Verification items for the finished model (mm, model axes). A direction names the side the tool comes from. Coordinates: 2 decimals unless noted, no trailing zeros. Order: outer loops, then holes, each group sorted by start corner. A loop starts at its lowest first (then second) coordinate and runs counter-clockwise, first axis right, second up. Notation, with made-up numbers: M 24.25,48.25 L 63.25,48.25 A7 cw 63.25,53.25 Z; hole C -19.75,4.5 d2. An arc over 180 degrees is marked long. Answer as a JSON object with one key per item and string values. Group by question number.
(1) Cross-section at D-D (y = 25). Enter the section's corners in (x, z), plus the area to 3 significant figures.
(2) Cross-section at C-C (z = 12.5). Enter the section's corners in (x, y), plus the area to 3 significant figures.
(3) Material ranges on line 1 (X direction, y = 0, z = 13.25); line 2 (Y direction, x = 0, z = 19.25); line 3 (X direction, y = -31.5, z = 22), recorded low to high.
(4) Cross-section at B-B (y = 0). Enter the section's corners in (x, z), plus the area to 3 significant figures.
(5) Cross-section at A-A (x = 0). Enter the section's corners in (y, z).
(6) Gauge pin test, flat ends, axial feed: pin 1 Ø0.8 at (y, z) = (-27, 22) entering from +X; pin 2 Ø4 at (x, y) = (-2, -31.5) entering from +Z. Record the tip position at first contact, or that the pin passes through.
(7) Mould release check, pull along Z, two halves, no side actions. Record for faces 4 (the face through (-32, 1, 25)), 5 (the face through (-63.5, -1, 12)), 6 (the face through (30.304, -0.533, 22.496)), 7 (the face through (38, -1, 19.92)): released by +Z, released by -Z, zero draft, split by the parting line, or undercut.
(8) Access from +Z, -Z, +X, -X, +Y, -Y to the whole of each face (thin tool, end or side, straight path). Record for faces 1 (the face through (-1, -38.1, 12)), 2 (the face through (68.509, -0.992, 20.055)), 3 (the face through (-54.61, -1, 22)).
from build123d import *

# Parameters (mm, degrees)
F0_W     = 127
F0_H     = 76.2
F0_R     = 20
F1_DEPTH = 25
F2_W     = 6.35
F2_H     = 76.2
F3_DEPTH = 5.08
F5_DEPTH = 76.201
F6_R     = 7.62
F7_DEPTH = 12.7
F8_R     = 2.54
F9_SIZE  = 2.54


with BuildPart() as f1:
    # F0 (on Top) → F1 (new body)
    with BuildSketch(Plane.XY):
        Rectangle(F0_W, F0_H)
        Circle(F0_R, mode=Mode.SUBTRACT)
    extrude(amount=F1_DEPTH)

    # F2 (on face) → F3 (cut)
    with BuildSketch(Plane.XY.offset(25)):
        with Locations((-57.785, 0)):
            Rectangle(F2_W, F2_H)
        with BuildLine():
            Line((-6.35, -18.9651654356), (-6.35, -38.1))
            Line((-6.35, -38.1), (6.35, -38.1))
            Line((6.35, -38.1), (6.35, -18.9651654356))
            ThreePointArc((6.35, -18.9651654356), (0, -20), (-6.35, -18.9651654356))
        make_face()
        with BuildLine():
            Line((6.35, 38.1), (-6.35, 38.1))
            Line((-6.35, 38.1), (-6.35, 18.9651654356))
            ThreePointArc((-6.35, 18.9651654356), (0, 20), (6.35, 18.9651654356))
            Line((6.35, 18.9651654356), (6.35, 38.1))
        make_face()
    extrude(amount=-F3_DEPTH, mode=Mode.SUBTRACT)

    # F4 (on face) → F5 (cut, through all)
    with BuildSketch(Plane.XZ.offset(38.1)):
        Polygon((44.45, 25), (31.75, 25), (28.8170606325, 19.92), (47.3829393675, 19.92), align=None)
    extrude(amount=-F5_DEPTH, mode=Mode.SUBTRACT)

    # F6 (on face) → F7 (join)
    with BuildSketch(Plane.YZ.offset(63.5)):
        with Locations((0, 12.5)):
            Circle(F6_R)
    extrude(amount=F7_DEPTH)

    # F8
    f8_edges = [f1.edges().sort_by_distance(p)[0] for p in [
        (-6.35, -28.532583, 25),
        (-6.35, 28.532583, 25),
        (6.35, 28.532583, 25),
        (6.35, -28.532583, 25),
    ]]
    fillet(f8_edges, radius=F8_R)

    # F9
    f9_edges = [f1.edges().sort_by_distance(p)[0] for p in [
        (76.2, -7.62, 12.5),
    ]]
    chamfer(f9_edges, length=F9_SIZE)


solid = f1.part
Taken from the geometry:
{
 "1": {"outline": "M -63.5,0 L 63.5,0 L 63.5,25 L 44.45,25 L 47.38,19.92 L 28.82,19.92 L 31.75,25 L 8.89,25 A2.54 ccw 6.35,22.46 L 6.35,19.92 L -6.35,19.92 L -6.35,22.46 A2.54 ccw -8.89,25 L -54.61,25 L -54.61,19.92 L -60.96,19.92 L -60.96,25 L -63.5,25 Z", "area": "3,000 mm²"},
 "2": {"outline": "M -63.5,-38.1 L 63.5,-38.1 L 63.5,-7.62 L 73.66,-7.62 L 76.2,-5.08 L 76.2,5.08 L 73.66,7.62 L 63.5,7.62 L 63.5,38.1 L -63.5,38.1 Z; hole C 0,0 d40", "area": "8,610 mm²"},
 "3": {"line 1": "x = -63.5 to -20, 20 to 76.2", "line 2": "y = -38.1 to -20, 20 to 38.1", "line 3": "x = -63.5 to -60.96, -54.61 to -6.35, 6.35 to 30.02, 46.18 to 63.5"},
 "4": {"outline": "M -63.5,0 L -20,0 L -20,25 L -54.61,25 L -54.61,19.92 L -60.96,19.92 L -60.96,25 L -63.5,25 Z; M 20,0 L 63.5,0 L 63.5,4.88 L 73.66,4.88 L 76.2,7.42 L 76.2,17.58 L 73.66,20.12 L 63.5,20.12 L 63.5,25 L 44.45,25 L 47.38,19.92 L 28.82,19.92 L 31.75,25 L 20,25 Z", "area": "2,250 mm²"},
 "5": {"outline": "M -38.1,0 L -20,0 L -20,19.92 L -38.1,19.92 Z; M 20,0 L 38.1,0 L 38.1,19.92 L 20,19.92 Z"},
 "6": {"pin 1": "stops at x = 63.5", "pin 2": "stops at z = 19.92"},
 "7": {"face 4": "released by +Z", "face 5": "zero draft", "face 6": "undercut", "face 7": "undercut"},
 "8": {"face 1": "+Z, -Z, +X, -X, -Y", "face 2": "+X", "face 3": "+Z, +Y, -Y"}
}
